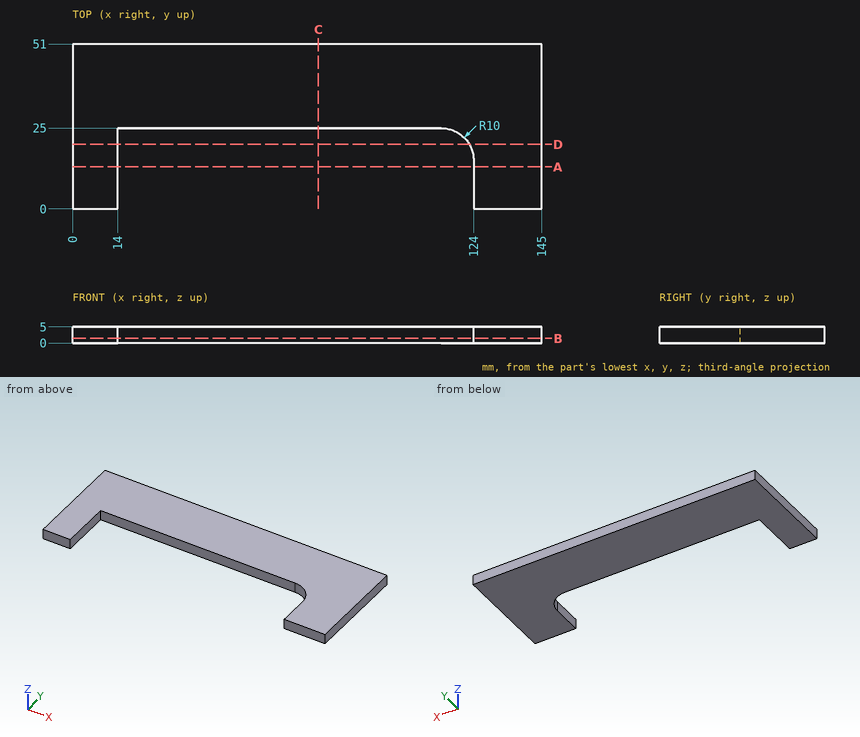
Verification items for this drawing (mm, ordinates from the low corner). Coordinates: 2 decimals unless noted, no trailing zeros. Loops run counter-clockwise (first coordinate to the right, second up) from the corner with the lowest first, then second, coordinate; pieces in that order, holes last. Notation, with made-up numbers: (-27, 9.25) - (-13, 9.25) arc R25 cw to (-13, 40.25) - close; hole circle Ø3 at (54.25, -24.5). An arc over 180 degrees is marked (long way). One line per item, written item: value. Start each with the question number.
(1) Cross-section at B-B on z = 1.5. Enter the section's corners in (x, y), plus the area to 3 significant figures.
(2) Material ranges on line 1 (X direction, y = 12.5, z = 1.9); line 2 (Y direction, x = 41, z = 4.65); line 3 (X direction, y = 18, z = 2.1), recorded low to high. Write a range as [from, to].
(3) Depth check by flat-ended pin: P1, Ø2.5, axis at x = 52, z = 1.5, coming from the -Y side. Enter the tip coordinate at first touch or a pass-through.
(4) Cross-section at C-C on x = 76. Enter the section's corners in (y, z), plus the area to 3 significant figures.
(5) Cross-section at D-D on y = 20. Enter the section's corners in (x, z).
(6) Cross-section at A-A on y = 13. Enter the section's corners in (x, z).
Results below:
1. outline: (0, 0) - (14, 0) - (14, 25) - (114, 25) arc R10 cw to (124, 15) - (124, 0) - (145, 0) - (145, 51) - (0, 51) - close
1. area: 4,670 mm2
2. line 1: x = [0, 14], [124, 145]
2. line 2: y = [25, 51]
2. line 3: x = [0, 14], [123.54, 145]
3. P1: stops at y = 25
4. outline: (25, 0) - (51, 0) - (51, 5) - (25, 5) - close
4. area: 130 mm2
5. outline: (0, 0) - (14, 0) - (14, 5) - (0, 5) - close; (122.66, 0) - (145, 0) - (145, 5) - (122.66, 5) - close
6. outline: (0, 0) - (14, 0) - (14, 5) - (0, 5) - close; (124, 0) - (145, 0) - (145, 5) - (124, 5) - close
